Autodesk Inventor part; units mm, degrees
ref_plane "BoardFrontPlane" through (0, 0, 0) normal (0, 0, 1) x (1, 0, 0)
ref_plane "YZ Plane" through (0, 0, 0) normal (1, 0, 0) x (0, 1, 0)
ref_plane "XZ Plane" through (0, 0, 0) normal (0, 1, 0) x (-1, 0, 0)
ref_plane "BoardFrontPlane" through (0, 0, 0) normal (0, 0, 1) x (1, 0, 0)
sketch "Sketch1" plane through (0, 0, 0) normal (0, 0, 1) x (1, 0, 0)
  line L0 (27.9236, 28.9773) -> (27.9236, 77.9773)
  line L1 (27.9236, 77.9773) -> (65.9236, 77.9773)
  line L2 (65.9236, 77.9773) -> (65.9236, 28.9773)
  line L3 (65.9236, 28.9773) -> (27.9236, 28.9773)
extrude "BoardOutline" add sketch "Sketch1" along normal blind 1.594
sketch "img_Top" plane through (0, 0, 1.594) normal (0, 0, 1) x (1, 0, 0)
  line L0 (27.9236, 77.9773) -> (65.9246, 77.9773) construction
  line L1 (65.9246, 77.9773) -> (65.9246, 28.9773) construction
  line L2 (65.9246, 28.9773) -> (27.9236, 28.9773) construction
  line L3 (27.9236, 28.9773) -> (27.9236, 77.9773) construction
decal "Decal_Top"
sketch "img_Bottom" plane through (0, 0, -1.594) normal (0, 0, -1) x (1, 0, 0)
  line L0 (27.9236, -28.9773) -> (65.9246, -28.9773) construction
  line L1 (65.9246, -28.9773) -> (65.9246, -77.9773) construction
  line L2 (65.9246, -77.9773) -> (27.9236, -77.9773) construction
  line L3 (27.9236, -77.9773) -> (27.9236, -28.9773) construction
decal "Decal_Bottom"
sketch "Sketch4" plane through (0, 0, 1.594) normal (0, 0, 1) x (1, 0, 0)
  point P0 (62.94, 42.86)
hole "Free-18" at (62.94, 42.86, 1.594) direction (0, 0, -1) diameter 3.2639 end through all
sketch "Sketch5" plane through (0, 0, 1.594) normal (0, 0, 1) x (1, 0, 0)
  point P0 (30.94, 42.86)
hole "Free-19" at (30.94, 42.86, 1.594) direction (0, 0, -1) diameter 3.2639 end through all
sketch "Sketch6" plane through (0, 0, 1.594) normal (0, 0, 1) x (1, 0, 0)
  point P0 (62.94, 75.21)
hole "Free-17" at (62.94, 75.21, 1.594) direction (0, 0, -1) diameter 3.2639 end through all
sketch "Sketch7" plane through (0, 0, 1.594) normal (0, 0, 1) x (1, 0, 0)
  point P0 (30.94, 75.21)
hole "Free-16" at (30.94, 75.21, 1.594) direction (0, 0, -1) diameter 3.2639 end through all
properties part number "nanobox_v31_upgrade_BOARD"
Part model, mm, in its own coordinate system. Coordinates: 2 decimals unless noted, no trailing zeros. Write each loop counter-clockwise with the first axis right and the second up, starting at its lowest first coordinate (ties: lowest second). Pieces come first, ordered by that corner, then holes.
Item 1: Mould opens along Y. For faces 1 (the face through (47, 28.977, 1)), 2 (the face through (47, 54, 1.594)), 3 (the face through (29.32, 43.07, 0.79)) say: released by +Y, released by -Y, zero draft, split by the parting line, or undercut.
Item 2: Slice it at A-A (x = 30.94). Write the cut outline in (y, z).
Item 3: Pin check, flat tip, straight feed: pin 1 (4 mm diameter, centred on x = 30.94, y = 75.21, fed in from -Z). Stop position of the tip, or through.
Item 4: Slice it at C-C (z = 1). Write the cut outline in (x, y), and give its area (3 significant figures).
Item 5: Probe line 1 (X direction, y = 75.21, z = 0.45); line 2 (Y direction, x = 62.94, z = 1.25); line 3 (Y direction, x = 30.5, z = 0.9). List the from-to ranges inside material, lowest first.
Item 6: Slice it at B-B (y = 42.86). Write the cut outline in (x, z).
Results found:
1. face 1: released by -Y
1. face 2: zero draft
1. face 3: undercut
2. outline: (28.98, 0) - (41.23, 0) - (41.23, 1.59) - (28.98, 1.59) - close; (44.49, 0) - (73.58, 0) - (73.58, 1.59) - (44.49, 1.59) - close; (76.84, 0) - (77.98, 0) - (77.98, 1.59) - (76.84, 1.59) - close
3. pin 1: stops at z = 0
4. outline: (27.92, 28.98) - (65.92, 28.98) - (65.92, 77.98) - (27.92, 77.98) - close; hole circle Ø3.26 at (30.94, 42.86); hole circle Ø3.26 at (30.94, 75.21); hole circle Ø3.26 at (62.94, 42.86); hole circle Ø3.26 at (62.94, 75.21)
4. area: 1,830 mm2
5. line 1: x = 27.92 to 29.31, 32.57 to 61.31, 64.57 to 65.92
5. line 2: y = 28.98 to 41.23, 44.49 to 73.58, 76.84 to 77.98
5. line 3: y = 28.98 to 41.29, 44.43 to 73.64, 76.78 to 77.98
6. outline: (27.92, 0) - (29.31, 0) - (29.31, 1.59) - (27.92, 1.59) - close; (32.57, 0) - (61.31, 0) - (61.31, 1.59) - (32.57, 1.59) - close; (64.57, 0) - (65.92, 0) - (65.92, 1.59) - (64.57, 1.59) - close
